from build123d import *

# Parameters (mm, degrees)
F0_R     = 6.35
F1_DEPTH = 11.43
F2_DEPTH = 14.986
F3_R     = 2.54


with BuildPart() as f1:
    # F0 (on Top) → F1 (new body)
    with BuildSketch(Plane.XY):
        with BuildLine():
            ThreePointArc((4.7624999017, -8.2488920278), (8.2488919427, -4.7625000491), (9.525, 0))
            ThreePointArc((9.525, 0), (8.2488920139, 4.7624999258), (4.7625001484, 8.2488918854))
            ThreePointArc((4.7625001484, 8.2488918854), (2.371e-07, 9.525), (-4.7624997378, 8.2488921224))
            ThreePointArc((-4.7624997378, 8.2488921224), (-8.2488918954, 4.7625001311), (-9.525, 0))
            ThreePointArc((-9.525, 0), (-8.2488919427, -4.7625000491), (-4.7624999017, -8.2488920278))
            ThreePointArc((-4.7624999017, -8.2488920278), (0, -9.525), (4.7624999017, -8.2488920278))
        make_face()
        Circle(F0_R, mode=Mode.SUBTRACT)
        with BuildLine():
            ThreePointArc((-9.525, 0), (-8.2488918954, 4.7625001311), (-4.7624997378, 8.2488921224))
            Line((-4.7624997378, 8.2488921224), (-9.525, 5.499261314))
            Line((-9.525, 5.499261314), (-9.525, 0))
        make_face()
        with BuildLine():
            ThreePointArc((-4.7624997378, 8.2488921224), (2.371e-07, 9.525), (4.7625001484, 8.2488918854))
            Line((4.7625001484, 8.2488918854), (0, 10.9985226281))
            Line((0, 10.9985226281), (-4.7624997378, 8.2488921224))
        make_face()
        with BuildLine():
            ThreePointArc((4.7625001484, 8.2488918854), (8.2488920139, 4.7624999258), (9.525, 0))
            Line((9.525, 0), (9.525, 5.499261314))
            Line((9.525, 5.499261314), (4.7625001484, 8.2488918854))
        make_face()
        with BuildLine():
            Line((9.525, -5.499261314), (9.525, 0))
            ThreePointArc((9.525, 0), (8.2488919427, -4.7625000491), (4.7624999017, -8.2488920278))
            Line((4.7624999017, -8.2488920278), (9.525, -5.499261314))
        make_face()
        with BuildLine():
            Line((0, -10.9985226281), (4.7624999017, -8.2488920278))
            ThreePointArc((4.7624999017, -8.2488920278), (0, -9.525), (-4.7624999017, -8.2488920278))
            Line((-4.7624999017, -8.2488920278), (0, -10.9985226281))
        make_face()
        with BuildLine():
            Line((-9.525, -5.499261314), (-4.7624999017, -8.2488920278))
            ThreePointArc((-4.7624999017, -8.2488920278), (-8.2488919427, -4.7625000491), (-9.525, 0))
            Line((-9.525, 0), (-9.525, -5.499261314))
        make_face()
    extrude(amount=F1_DEPTH)

    # F0 (on Top) → F2 (join)
    with BuildSketch(Plane.XY):
        with BuildLine():
            ThreePointArc((4.7624999017, -8.2488920278), (8.2488919427, -4.7625000491), (9.525, 0))
            ThreePointArc((9.525, 0), (8.2488920139, 4.7624999258), (4.7625001484, 8.2488918854))
            ThreePointArc((4.7625001484, 8.2488918854), (2.371e-07, 9.525), (-4.7624997378, 8.2488921224))
            ThreePointArc((-4.7624997378, 8.2488921224), (-8.2488918954, 4.7625001311), (-9.525, 0))
            ThreePointArc((-9.525, 0), (-8.2488919427, -4.7625000491), (-4.7624999017, -8.2488920278))
            ThreePointArc((-4.7624999017, -8.2488920278), (0, -9.525), (4.7624999017, -8.2488920278))
        make_face()
        Circle(F0_R, mode=Mode.SUBTRACT)
    extrude(amount=F2_DEPTH)

    # F3
    f3_edges = [f1.edges().sort_by_distance(p)[0] for p in [
        (-9.525, 0, 14.986),
    ]]
    fillet(f3_edges, radius=F3_R)


solid = f1.part
Model file for the job. Use its own axes, mm. A direction names the side the tool comes from. Coordinates: 2 decimals unless noted, no trailing zeros. Use one line per item in the form item = value. Start each with the question number.
(1) Tool access for faces 3 (the flat face through (-9, 5, 11.43)), 4 (the flat face through (9, 5, 11.43)), 5 (the flat face through (9, -5, 11.43)), 6 (the flat face through (0, -10, 11.43)): list every direction of +Z, -Z, +X, -X, +Y, -Y with a clear straight run to the whole face (end or side of a thin tool).
(2) Pull direction Y, two halves, no side cores. Call faces 1 (the flat face through (3, -6, 14.986)), 2 (the cylindrical face through (-1.38, -6.2, 7.39)): pulls with the +Y half, pulls with the -Y half, needs draft (parallel to the pull), parting line crosses it, or undercut.
(3) Flat gauge pins, fed straight in: pin 1 (2 mm diameter, centred on x = -2, y = -9.5, fed in from +Z); pin 2 (5 mm diameter, centred on x = -7.5, z = 7.5, fed in from -Y); pin 3 (1.5 mm diameter, centred on x = 6, z = 10.5, fed in from -Y). Where does each tip first touch, or does it go through?
(4) Probe probe 1 along Y at (x, z) = (-3.75, 3.25); probe 2 along Y at (x, z) = (-4.75, 11.25); probe 3 along X at (y, z) = (-4, 8) (3 decimals). List the from-to ranges inside material, lowest first. Write a range as from..to.
Values:
q1.face_3 = +Z, -X, +Y
q1.face_4 = +Z, +X, +Y
q1.face_5 = +Z, +X, -Y
q1.face_6 = +Z, -Y
q2.face_1 = needs draft
q2.face_2 = undercut
q3.pin_1 = 14.31
q3.pin_2 = -8.11
q3.pin_3 = -7.97
q4.probe_1 = -8.83..-5.12, 5.12..8.83
q4.probe_2 = -8.26..-4.21, 4.21..8.26
q4.probe_3 = -9.525..-4.932, 4.932..9.525
